```python
from build123d import *

# Parameters (mm, degrees)
CHAMFER1_SIZE      = 0.5
CHAMFER2_SIZE      = 0.3
CUT_EXTRUDE1_DEPTH = 2.5
CHAMFER3_SIZE      = 0.3


with BuildPart() as part:
    # Sketch1 → Revolve1 (revolve)
    with BuildSketch(Plane.XY):
        Polygon((0, 0), (0, 2.75), (3, 2.75), (3, 1.49), (15, 1.49), (15, 0), align=None)
    revolve(axis=Axis((-88.705490849, 0, 0), (1, 0, 0)))

    # Chamfer1
    chamfer1_edges = [part.edges().sort_by_distance(p)[0] for p in [
        (15, -1.49, 0),
    ]]
    chamfer(chamfer1_edges, length=CHAMFER1_SIZE)

    # Chamfer2
    chamfer2_edges = [part.edges().sort_by_distance(p)[0] for p in [
        (0, -2.75, 0),
    ]]
    chamfer(chamfer2_edges, length=CHAMFER2_SIZE)

    # Sketch3 → Cut-Extrude1 (cut)
    with BuildSketch(Plane(origin=(0, 0, 0), x_dir=(0, 0, -1), z_dir=(1, 0, 0))):
        Polygon((-1.443375673, 0), (-0.721687836, -1.25), (0.721687836, -1.25), (1.443375673, 0), (0.721687836, 1.25), (-0.721687836, 1.25), align=None)
    extrude(amount=CUT_EXTRUDE1_DEPTH, mode=Mode.SUBTRACT)

    # Chamfer3
    chamfer3_edges = [part.edges().sort_by_distance(p)[0] for p in [
        (0, 0.625, 1.082531755),
        (0, -0.625, 1.082531755),
        (0, -1.25, 0),
        (0, -0.625, -1.082531755),
        (0, 0.625, -1.082531755),
        (0, 1.25, 0),
    ]]
    chamfer(chamfer3_edges, length=CHAMFER3_SIZE)


solid = part.part
```
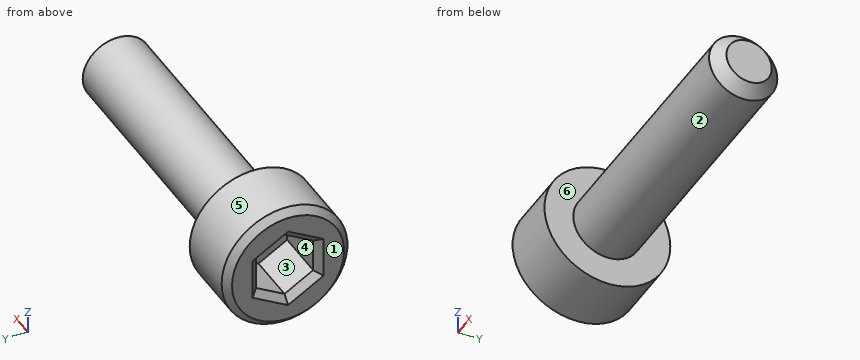
Read the model definition and answer for the solid it produces. Units are mm, in the model's axes. Face numbers are marked on the shaded views. A direction names the side the tool comes from. Give positions to 0.01 mm unless a question says otherwise; leave off trailing zeros. Order: outer loops, then holes, each group sorted by start corner. A loop starts at its lowest first (then second) coordinate and runs counter-clockwise, first axis right, second up.
(1) Find section B-B (x = 4.25). Give the vertices of the cut face in (y, z).
(2) For a pull along Z with two mould halves and no side action, classify the marked faces 4, 5 and 6 as released by +Z, released by -Z, zero draft, split by the parting line, or undercut.
(3) For the marked faces 1, 2 and 3, determine the directions among +Z, -Z, +X, -X, +Y, -Y from which every point of the face is accessible in a straight line to the end or side of a thin tool.
(4) Given pin 1 (1.5 mm diameter, centred on x = 7, y = -1, fed in from +Z); pin 2 (1 mm diameter, centred on x = 4.5, z = -1.5, fed in from -Y); pin 3 (1 mm diameter, centred on x = 9, z = -1, fed in from -Y); pin 4 (3 mm diameter, centred on y = -0.5, z = -0.5, fed in from -X), each flat-ended and moving along its own axis, determine where each tip first touches the part or whether it passes through.
(5) Find section A-A (z = 0). Give the vertices of the cut face in (x, y), plus the area to 3 significant figures.
(6) Straight lines are drawn through the part: L1, parallel to X at y = -1.85, z = -0.6; L2, parallel to Y at x = 1, z = 1.05; L3, parallel to Y at x = 5.5, z = 0.05. For each, find the intervals that lie inside material, in ascending order.
Result sheet:
1. outline: circle Ø2.98 at (0, 0)
2. face 4: undercut
2. face 5: split by the parting line
2. face 6: zero draft
3. face 1: +Z, -Z, -X, +Y, -Y
3. face 2: +X
3. face 3: -X
4. pin 1: stops at z = 1.47
4. pin 2: stops at y = -1.1
4. pin 3: stops at y = -1.4
4. pin 4: stops at x = 0
5. outline: (0, -2.45) - (0.3, -2.75) - (3, -2.75) - (3, -1.49) - (14.5, -1.49) - (15, -0.99) - (15, 0.99) - (14.5, 1.49) - (3, 1.49) - (3, 2.75) - (0.3, 2.75) - (0, 2.45) - (0, 1.55) - (0.3, 1.25) - (2.5, 1.25) - (2.5, -1.25) - (0.3, -1.25) - (0, -1.55) - close
5. area: 45.6 mm2
6. L1: x = 0 to 3
6. L2: y = -2.54 to -0.68, 0.68 to 2.54
6. L3: y = -1.49 to 1.49
